```python
from build123d import *

# Parameters (mm, degrees)
BOSS_EXTRUDE1_DEPTH     = 2
SKETCH2_R               = 3.2
SKETCH2_R_2             = 3.25
CUT_HOLES_DEPTH         = 3
CUT_HOLES_DEPTH_BACK    = 3
SKETCH3_R               = 13.5
SKETCH3_W               = 19
SKETCH3_H               = 36
CUT_EXTRUDE2_DEPTH      = 3
CUT_EXTRUDE2_DEPTH_BACK = 3


with BuildPart() as part:
    # Sketch1 → Boss-Extrude1 (new body, symmetric)
    with BuildSketch(Plane(origin=(0, 0, 0), x_dir=(1, 0, 0), z_dir=(0, 1, 0))):
        with BuildLine():
            Line((86.2, 39.931942102), (86.2, -39.931942102))
            ThreePointArc((86.2, -39.931942102), (0, -81.597763245), (-86.2, -39.931942102))
            Line((-86.2, -39.931942102), (-86.2, 39.931942102))
            ThreePointArc((-86.2, 39.931942102), (0, 95), (86.2, 39.931942102))
        make_face()
    extrude(amount=BOSS_EXTRUDE1_DEPTH, both=True)

    # Sketch2 → Cut-Holes (cut, two sides)
    with BuildSketch(Plane(origin=(0, 0, 0), x_dir=(1, 0, 0), z_dir=(0, 1, 0))) as cut_holes_sk:
        with Locations((-75, 10.7)):
            Circle(SKETCH2_R)
        with Locations((-75, -40.7)):
            Circle(SKETCH2_R)
        with Locations((75, -40.7)):
            Circle(SKETCH2_R)
        with Locations((75, 10.7)):
            Circle(SKETCH2_R)
        with Locations((0, -71.597763245)):
            Circle(SKETCH2_R_2)
        with Locations((0, 85)):
            Circle(SKETCH2_R_2)
        with Locations((-75.036257902, 39.931942102)):
            Circle(SKETCH2_R_2)
        with Locations((75.036257902, 39.931942102)):
            Circle(SKETCH2_R_2)
        with BuildLine():
            ThreePointArc((14.471626034, -67.259325745), (11.744315506, -70.958890218), (15.443879979, -73.686200745))
            ThreePointArc((15.443879979, -73.686200745), (40.475581865, -66.58349782), (62.936747266, -53.448409812))
            ThreePointArc((62.936747266, -53.448409812), (63.532100029, -48.890937367), (58.974627584, -48.295584605))
            ThreePointArc((58.974627584, -48.295584605), (37.92748228, -60.603766345), (14.471626034, -67.259325745))
        make_face()
        with BuildLine():
            ThreePointArc((-62.936747266, -53.448409812), (-63.532100029, -48.890937367), (-58.974627584, -48.295584605))
            ThreePointArc((-58.974627584, -48.295584605), (-37.92748228, -60.603766345), (-14.471626034, -67.259325745))
            ThreePointArc((-14.471626034, -67.259325745), (-11.744315506, -70.958890218), (-15.443879979, -73.686200745))
            ThreePointArc((-15.443879979, -73.686200745), (-40.475581865, -66.58349782), (-62.936747266, -53.448409812))
        make_face()
        with BuildLine():
            ThreePointArc((-63.94162293, 50.936542452), (-68.508644796, 50.419520904), (-69.025666344, 54.98654277))
            ThreePointArc((-69.025666344, 54.98654277), (-45.1765399, 75.809911903), (-15.512787354, 86.875865052))
            ThreePointArc((-15.512787354, 86.875865052), (-11.742100438, 84.24776304), (-14.37020245, 80.477076125))
            ThreePointArc((-14.37020245, 80.477076125), (-41.849089369, 70.226179015), (-63.94162293, 50.936542452))
        make_face()
        with BuildLine():
            ThreePointArc((15.512787354, 86.875865052), (11.742100438, 84.24776304), (14.37020245, 80.477076125))
            ThreePointArc((14.37020245, 80.477076125), (41.849089369, 70.226179015), (63.94162293, 50.936542452))
            ThreePointArc((63.94162293, 50.936542452), (68.508644796, 50.419520904), (69.025666344, 54.98654277))
            ThreePointArc((69.025666344, 54.98654277), (45.1765399, 75.809911903), (15.512787354, 86.875865052))
        make_face()
    extrude(amount=CUT_HOLES_DEPTH, mode=Mode.SUBTRACT)
    extrude(cut_holes_sk.sketch, amount=-CUT_HOLES_DEPTH_BACK, mode=Mode.SUBTRACT)

    # Sketch3 → Cut-Extrude2 (cut, two sides)
    with BuildSketch(Plane(origin=(0, 0, 0), x_dir=(1, 0, 0), z_dir=(0, 1, 0))) as cut_extrude2_sk:
        with Locations((0, 60)):
            Circle(SKETCH3_R)
        with Locations((-15.2, -15)):
            Rectangle(SKETCH3_W, SKETCH3_H)
        with Locations((15.2, -15)):
            Rectangle(SKETCH3_W, SKETCH3_H)
    extrude(amount=CUT_EXTRUDE2_DEPTH, mode=Mode.SUBTRACT)
    extrude(cut_extrude2_sk.sketch, amount=-CUT_EXTRUDE2_DEPTH_BACK, mode=Mode.SUBTRACT)


solid = part.part
```
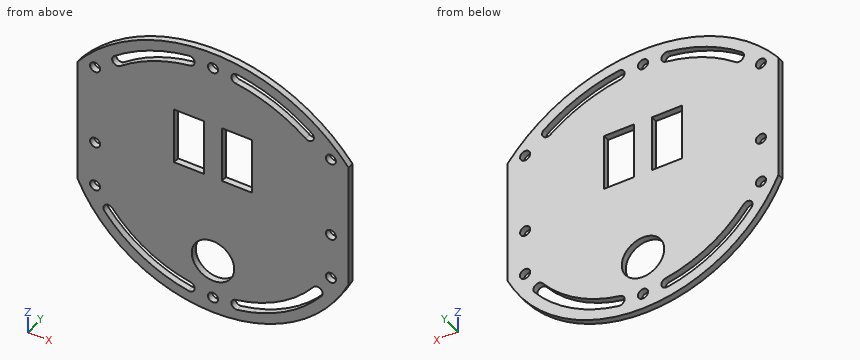
Work out the finished part from the listing and answer in its coordinate system (mm). Give positions to 0.01 mm unless a question says otherwise; leave off trailing zeros. Write each loop counter-clockwise with the first axis right and the second up, starting at its lowest first coordinate (ties: lowest second). Pieces come first, ordered by that corner, then holes. Notation, with made-up numbers: (27, -5.5) -> (32, -5.5) arc R12 ccw to (32, 11.5) -> close; hole circle Ø6 at (-27.75, 59.25). An arc over 180 degrees is marked (long way). Write each question's results on one line, items separated by ' | '.
1. Straight lines are drawn through the part: L1, parallel to Z at x = 0, y = 1.1; L2, parallel to X at y = 0.65, z = -60; L3, parallel to Z at x = 52.5, y = 0.65. For each, find the intervals that lie inside material, in ascending order.
Data:
L1: -95 to -88.25, -81.75 to -73.5, -46.5 to 68.35, 74.85 to 81.6 | L2: -73.65 to -64.72, -55.53 to -13.5, 13.5 to 55.53, 64.72 to 73.65 | L3: -79.18 to -70.94, -62.66 to 52.86, 60.5 to 68.26
2. Find section C-C on z = -53. Determine the outline of the cut face in (x, y), and give its area (3 significant figures).
Data:
outline: (-78.84, -2) -> (-69.73, -2) -> (-69.73, 2) -> (-78.84, 2) -> close; (-62.24, -2) -> (-11.54, -2) -> (-11.54, 2) -> (-62.24, 2) -> close; (11.54, -2) -> (62.24, -2) -> (62.24, 2) -> (11.54, 2) -> close; (69.73, -2) -> (78.84, -2) -> (78.84, 2) -> (69.73, 2) -> close | area: 478 mm^2
3. Find section D-D on x = 75. Determine the outline of the cut face in (y, z), and give its area (3 significant figures).
Data:
outline: (-2, -58.31) -> (2, -58.31) -> (2, -43.18) -> (-2, -43.18) -> close; (-2, -36.68) -> (2, -36.68) -> (2, -13.9) -> (-2, -13.9) -> close; (-2, -7.5) -> (2, -7.5) -> (2, 37.5) -> (-2, 37.5) -> close; (-2, 43.9) -> (2, 43.9) -> (2, 52.07) -> (-2, 52.07) -> close | area: 364 mm^2
4. Each of these flat-tipped pins is pushed along its axis until it touches: pin 1 Ø8.5 at (x, z) = (-75.04, -39.93) entering from -Y; pin 2 Ø2 at (x, y) = (-17.5, 0) entering from -Z; pin 3 Ø2 at (x, y) = (-53, 1) entering from -Z; pin 4 Ø1.2 at (x, y) = (12.5, 0.5) entering from -Z. Where does it stop, or does it pass through?
Data:
pin 1: y = -2 | pin 2: z = -93.56 | pin 3: z = -79.5 | pin 4: z = -94.25
5. Find section A-A on z = -10.7. Determine the outline of the cut face in (x, y), and give its area (3 significant figures).
Data:
outline: (-86.2, -2) -> (-78.2, -2) -> (-78.2, 2) -> (-86.2, 2) -> close; (-71.8, -2) -> (71.8, -2) -> (71.8, 2) -> (-71.8, 2) -> close; (78.2, -2) -> (86.2, -2) -> (86.2, 2) -> (78.2, 2) -> close | area: 638 mm^2
6. Find section B-B on x = -56. Determine the outline of the cut face in (y, z), and give its area (3 significant figures).
Data:
outline: (-2, -76.74) -> (2, -76.74) -> (2, -68.21) -> (-2, -68.21) -> close; (-2, -59.56) -> (2, -59.56) -> (2, 50.49) -> (-2, 50.49) -> close; (-2, 58.34) -> (2, 58.34) -> (2, 66.28) -> (-2, 66.28) -> close | area: 506 mm^2
